from build123d import *

# Parameters (mm, degrees)
F0_W      = 107.95
F0_H      = 63.5
F1_DEPTH  = 57.15
F2_W      = 31.75
F2_H      = 25.4
F3_DEPTH  = 107.951
F4_W      = 31.75
F4_H      = 12.7
F5_DEPTH  = 63.5
F6_W      = 50.8
F6_H      = 31.75
F7_DEPTH  = 25.4
F8_R      = 6.35
F9_DEPTH  = 31.751
F10_W     = 6.35
F10_H     = 6.35
F11_DEPTH = 63.501
F13_DEPTH = 31.751
F15_DEPTH = 57.151


with BuildPart() as f1:
    # F0 (on Top) → F1 (new body)
    with BuildSketch(Plane.XY):
        with Locations((53.975, 31.75)):
            Rectangle(F0_W, F0_H)
    extrude(amount=F1_DEPTH)

    # F2 (on face) → F3 (cut, through all)
    with BuildSketch(Plane(origin=(0, 0, 0), x_dir=(0, -1, 0), z_dir=(-1, 0, 0))):
        with Locations((-15.875, 44.45)):
            Rectangle(F2_W, F2_H)
    extrude(amount=-F3_DEPTH, mode=Mode.SUBTRACT)

    # F4 (on face) → F5 (cut)
    with BuildSketch(Plane.YZ.offset(107.95)):
        with Locations((15.875, 25.4)):
            Rectangle(F4_W, F4_H)
        with Locations((15.875, 6.35)):
            Rectangle(F4_W, F4_H)
    extrude(amount=-F5_DEPTH, mode=Mode.SUBTRACT)

    # F6 (on face) → F7 (cut)
    with BuildSketch(Plane.XY.offset(19.05)):
        with Locations((82.55, 15.875)):
            Rectangle(F6_W, F6_H)
    extrude(amount=-F7_DEPTH, mode=Mode.SUBTRACT)

    # F8 (on face) → F9 (cut, through all)
    with BuildSketch(Plane.XZ.offset(-31.75)):
        with Locations((19.05, 44.45)):
            Circle(F8_R)
    extrude(amount=-F9_DEPTH, mode=Mode.SUBTRACT)

    # F10 (on face) → F11 (cut, through all)
    with BuildSketch(Plane.XZ):
        with Locations((3.175, 3.175)):
            Rectangle(F10_W, F10_H)
    extrude(amount=-F11_DEPTH, mode=Mode.SUBTRACT)

    # F12 (on face) → F13 (cut, through all)
    with BuildSketch(Plane.XZ.offset(-31.75)):
        Polygon((107.95, 57.15), (44.45, 57.15), (107.95, 31.75), align=None)
    extrude(amount=-F13_DEPTH, mode=Mode.SUBTRACT)

    # F14 (on face) → F15 (cut, through all)
    with BuildSketch(Plane.XY):
        Polygon((82.55, 63.5), (107.95, 38.1), (107.95, 63.5), align=None)
    extrude(amount=F15_DEPTH, mode=Mode.SUBTRACT)


solid = f1.part
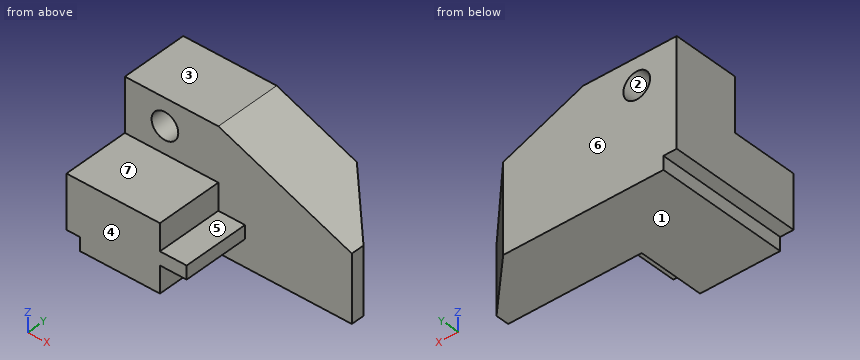
Design review of the part built by this model. Coordinates are the model's own, in mm. Face numbers are marked on the shaded views. A direction names the side the tool comes from. Round coordinates to 2 decimals unless told otherwise and drop trailing zeros. Write each loop counter-clockwise with the first axis right and the second up, starting at its lowest first coordinate (ties: lowest second). Pieces come first, ordered by that corner, then holes. Notation, with made-up numbers: (16.5, 81.5) - (40.5, 81.5) arc R22 cw to (40.5, 116.5) - close; hole circle Ø2 at (31, -20). An arc over 180 degrees is marked (long way). Return JSON: item names as keys, results as strings. Group by question number.
Item 1: Machinability: for the marked faces 5, 6 and 7, which of the approach directions +Z, -Z, +X, -X, +Y, -Y give a long, thin tool a straight path to every point of the face, cutting with its end or side? Answer none if there is none.
Item 2: For probe 1 along Z at (x, y) = (19.05, 57.5); probe 2 along Y at (x, z) = (27.5, 39); probe 3 along X at (y, z) = (8.5, 25), list the stretches that pass through material, from the lowest coordinate up. Write a range as [from, to].
Item 3: We need section B-B on x = 17.5. Write out the cut boundary in (y, z), and give its area (3 significant figures).
Item 4: Insertion check: P1, Ø7, axis at y = 22, z = 14.5, coming from the +X side; P2, Ø10, axis at y = 50, z = 35.5, coming from the +X side; P3, Ø6.5, axis at y = 22, z = 9, coming from the +X side; P4, Ø11.5, axis at x = 19.05, z = 44.45, coming from the +Y side. Each pin has a flat end and moves straight along its axis. Give the tip position at first contact, or say it passes through.
Item 5: The part is to be moulded in two halves that separate along Z. For the marked faces 1, 2, 3 and 4, say which applies: pulls with the +Z half, pulls with the -Z half, needs draft (parallel to the pull), parting line crosses it, or undercut.
Item 6: We need section A-A on z = 44.45. Write out the cut boundary in (x, y), and give its area (3 significant figures).
Item 7: We need section C-C on y = 57. Write out the cut boundary in (x, z).
Item 8: We need section D-D on z = 21. Write out the cut boundary in (x, y).
Model answer:
{
 "1": {"face 5": "+Z, +X, -Y", "face 6": "+Z, -Z, +X, -X, +Y", "face 7": "+Z, +X, -X, -Y"},
 "2": {"probe 1": "z = [0, 38.1], [50.8, 57.15]", "probe 2": "y = [31.75, 63.5]", "probe 3": "x = [0, 44.45]"},
 "3": {"outline": "(0, 0) - (63.5, 0) - (63.5, 38.29) - (31.75, 38.29) - (31.75, 31.75) - (0, 31.75) - close; (31.75, 50.61) - (63.5, 50.61) - (63.5, 57.15) - (31.75, 57.15) - close", "area": "2,430 mm²"},
 "4": {"P1": "stops at x = 57.15", "P2": "stops at x = 100.96", "P3": "stops at x = 44.45", "P4": "passes through"},
 "5": {"face 1": "pulls with the -Z half", "face 2": "undercut", "face 3": "pulls with the +Z half", "face 4": "needs draft"},
 "6": {"outline": "(0, 31.75) - (12.7, 31.75) - (12.7, 63.5) - (0, 63.5) - close; (25.4, 31.75) - (76.2, 31.75) - (76.2, 63.5) - (25.4, 63.5) - close", "area": "2,020 mm²"},
 "7": {"outline": "(0, 6.35) - (6.35, 6.35) - (6.35, 0) - (89.05, 0) - (89.05, 39.31) - (44.45, 57.15) - (0, 57.15) - close; hole circle Ø12.7 at (19.05, 44.45)"},
 "8": {"outline": "(0, 0) - (44.45, 0) - (44.45, 31.75) - (107.95, 31.75) - (107.95, 38.1) - (82.55, 63.5) - (0, 63.5) - close"}
}
